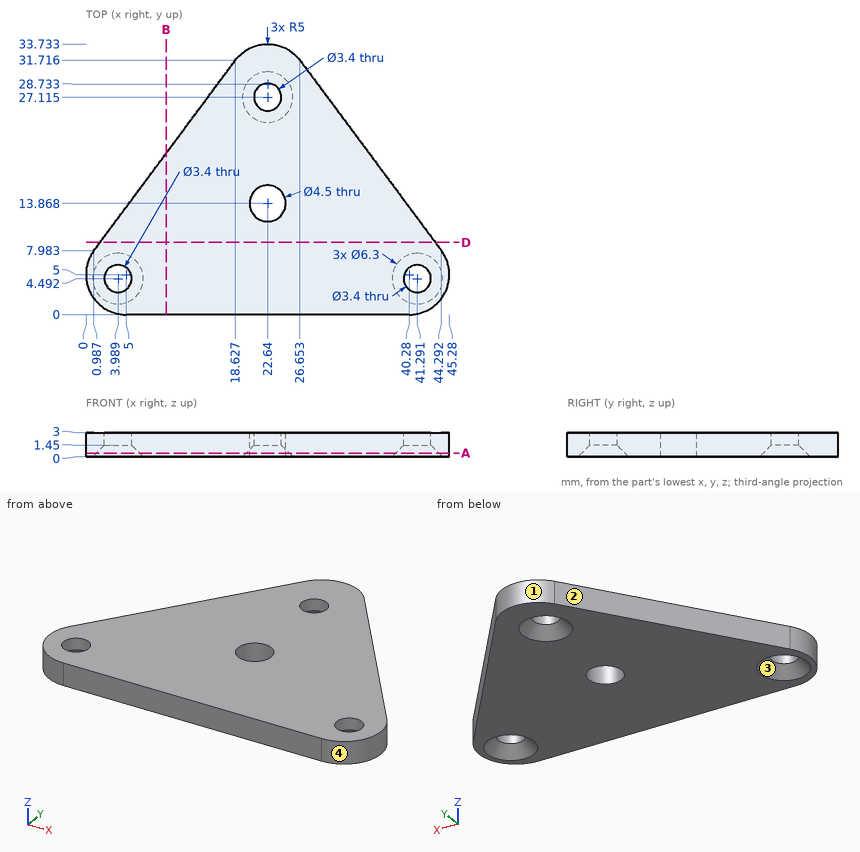
Design review of the part shown in the three views and the two pictorial views. Dimensions are in mm from the part's minimum x, y and z. Give positions to 0.01 mm unless a question says otherwise; leave off trailing zeros. Loops run counter-clockwise (first coordinate to the right, second up) from the corner with the lowest first, then second, coordinate; pieces in that order, holes last. Notation, with made-up numbers: (58.25, 2) -> (66.25, 2) arc R17 ccw to (66.25, 7) -> close; hole circle Ø8 at (44, -13.5). An arc over 180 degrees is marked (long way). One line per question, with ' | ' between items.
1) We need section A-A (z = 0.45). Give the number of separate pieces and of enclosed holes in the cut face.
Resolved:
separate pieces: 1 | enclosed holes: 4
2) We need section D-D (y = 9). Write out the cut boundary in (x, z), plus the area to 3 significant figures.
Resolved:
outline: (1.74, 0) -> (43.54, 0) -> (43.54, 3) -> (1.74, 3) -> close | area: 125 mm2
3) Insertion check: pin 1 Ø5.5 at (x, y) = (22.64, 27.12) entering from -Z (1 decimal); pin 2 Ø1 at (x, z) = (24, 1.5) entering from +Y. Each pin has a flat end and moves straight along its axis. Give the tip position at first contact, or say it passes through.
Resolved:
pin 1: stops at z = 0.4 | pin 2: stops at y = 33.66
4) We need section B-B (x = 10). Write out the cut boundary in (y, z).
Resolved:
outline: (0, 0) -> (20.11, 0) -> (20.11, 3) -> (0, 3) -> close
5) To check wall thickness, follow probe 1 along Y at (x, z) = (23, 0.5) (1 decimal); probe 2 along Y at (x, z) = (22, 0.5) (1 decimal); probe 3 along X at (y, z) = (6, 1.15) (1 decimal). State the ranges of each line that lie inside material, in increasing order.
Resolved:
probe 1: y = 0 to 11.6, 16.1 to 24.5, 29.7 to 33.7 | probe 2: y = 0 to 11.7, 16 to 24.5, 29.7 to 33.7 | probe 3: x = 0.1 to 2.7, 5.3 to 40, 42.6 to 45.2
6) The part is to be moulded in two halves that separate along X. For the marked faces 1, 2, 3 and 4, say which applies: +X half, -X half, draft (parallel to the pull), parting line (faces both ways), or undercut.
Resolved:
face 1: parting line | face 2: -X half | face 3: undercut | face 4: +X half
